```python
from build123d import *

# Parameters (mm, degrees)
SKETCH_1_R      = 7.5
EXTRUDE_1_DEPTH = 30
EXTRUDE_2_DEPTH = 9
EXTRUDE_START   = -15
EXTRUDE_3_DEPTH = 3.5


with BuildPart() as part:
    # Sketch 1 → Extrude 1 (new body)
    with BuildSketch(Plane(origin=(0, 0, 0), x_dir=(1, 0, 0), z_dir=(0, 1, 0))):
        with BuildLine():
            Line((14, -15), (0, -15))
            ThreePointArc((0, -15), (-15, 0), (0, 15))
            Line((0, 15), (14, 15))
            Line((14, 15), (14, -15))
        make_face()
        with Locations(Location((0, 0, 0), (0, 0, 270))):
            Circle(SKETCH_1_R, mode=Mode.SUBTRACT)
    extrude(amount=EXTRUDE_1_DEPTH)

    # Sketch 1_3 → Extrude 2 (add)
    with BuildSketch(Plane(origin=(0, 0, 0), x_dir=(1, 0, 0), z_dir=(0, 1, 0))):
        Polygon((14, 15), (14, -15), (46, -15), (55, -6), (55, 6), (46, 15), align=None)
    extrude(amount=EXTRUDE_2_DEPTH)

    # Sketch 2 → Extrude 3 (add, symmetric)
    with BuildSketch(Plane.XY.offset(15).offset(EXTRUDE_START)):
        Polygon((14, 30), (55, 9), (14, 9), align=None)
    extrude(amount=EXTRUDE_3_DEPTH, both=True)


solid = part.part
```
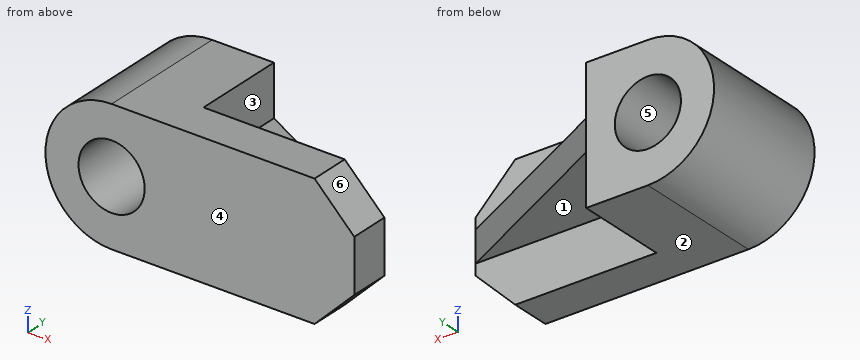
The model under review builds one solid part; all positions refer to its coordinate system, in mm. Face numbers are marked on the shaded views. A direction names the side the tool comes from. Round coordinates to 2 decimals unless told otherwise and drop trailing zeros. Loops run counter-clockwise (first coordinate to the right, second up) from the corner with the lowest first, then second, coordinate; pieces in that order, holes last. Notation, with made-up numbers: (77.5, 70.25) -> (122.5, 70.25) arc R25 cw to (122.5, 101.25) -> close; hole circle Ø4 at (15.25, 10). An arc over 180 degrees is marked (long way). Answer as a JSON object with one key per item and string values. Group by question number.
1) For pin 1 Ø4 at (y, z) = (25.5, 4.5) entering from -X; pin 2 Ø6 at (x, z) = (43, 7.5) entering from +Y; pin 3 Ø6 at (y, z) = (15.5, 7) entering from +X; pin 4 Ø13.5 at (x, z) = (0, 0) entering from +Y, all flat-tipped, find the tip position at first contact; note any pin that passes through.
2) For the marked faces 1, 2 and 3, list the 3-axis set-ups (+Z, -Z, +X, -X, +Y, -Y) from which the entire face can be reached by the end or side of a thin tool; tool diameter is ignored.
3) We need section B-B on y = 7. Write out the cut boundary in (x, z).
4) We need section C-C on z = -9. Write out the cut boundary in (x, y), then the cut area to 3 significant figures.
5) For line 1 (X direction, y = 6, z = 0); line 2 (Y direction, x = 20, z = -12); line 3 (X direction, y = 5.75, z = -3.75), list the stretches that pass through material, from the lowest coordinate up. Write a range as [from, to].
6) Mouldability with a two-part tool opening along Z and no side actions: class the marked faces 4, 5 and 6 as released by +Z, released by -Z, zero draft, split by the parting line, or undercut.
7) We need section D-D on y = 15. Write out the cut boundary in (x, z), then the cut area to 3 significant figures.
8) We need section A-A on z = 0. Write out the cut boundary in (x, y), then the cut area to 3 significant figures.
Result set:
{
 "1": {"pin 1": "x = -14.79", "pin 2": "y = 9", "pin 3": "x = 14", "pin 4": "through"},
 "2": {"face 1": "-Z, +X, +Y", "face 2": "-Z, +X, -X, +Y, -Y", "face 3": "+Z, +X, +Y"},
 "3": {"outline": "(0, -15) -> (46, -15) -> (55, -6) -> (55, 6) -> (46, 15) -> (0, 15) arc R15 ccw to start; hole circle Ø15 at (0, 0)"},
 "4": {"outline": "(-12, 0) -> (52, 0) -> (52, 9) -> (14, 9) -> (14, 30) -> (-12, 30) -> close", "area": "1,120 mm²"},
 "5": {"line 1": "[-15, -7.5], [7.5, 55]", "line 2": "[0, 9]", "line 3": "[-14.52, -6.5], [6.5, 55]"},
 "6": {"face 4": "zero draft", "face 5": "undercut", "face 6": "released by +Z"},
 "7": {"outline": "(0, -15) -> (14, -15) -> (14, -3.5) -> (43.29, -3.5) -> (43.29, 3.5) -> (14, 3.5) -> (14, 15) -> (0, 15) arc R15 ccw to start; hole circle Ø15 at (0, 0)", "area": "802 mm²"},
 "8": {"outline": "(-15, 0) -> (-7.5, 0) -> (-7.5, 30) -> (-15, 30) -> close; (7.5, 0) -> (55, 0) -> (55, 9) -> (14, 30) -> (7.5, 30) -> close", "area": "1,220 mm²"}
}
